Geometry check sheet. Reference: the model listing, model coordinates, mm. Face numbers are marked on the shaded views. Round coordinates to 2 decimals unless told otherwise and drop trailing zeros. Order: outer loops, then holes, each group sorted by start corner. A loop starts at its lowest first (then second) coordinate and runs counter-clockwise, first axis right, second up.
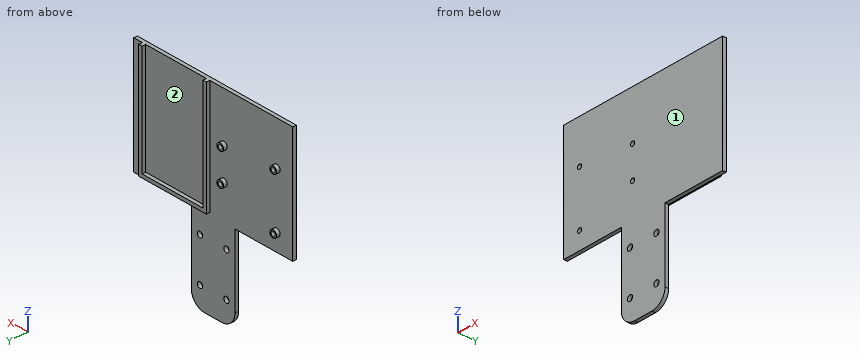
```python
from build123d import *

# Parameters (mm, degrees)
SKETCH1_W           = 41.91
SKETCH1_H           = 76.2
SKETCH1_R           = 2.54
BOSS_EXTRUDE1_DEPTH = 3.175
SKETCH2_W           = 152.4
SKETCH2_H           = 101.6
BOSS_EXTRUDE2_DEPTH = 3.175
SKETCH3_R           = 2
CUT_EXTRUDE1_DEPTH  = 160.162214816
BOSS_EXTRUDE3_DEPTH = 3.175
BOSS_EXTRUDE4_START = 3.175
SKETCH5_R           = 3.175
SKETCH5_R_2         = 2
BOSS_EXTRUDE4_DEPTH = 3.175
FILLET1_R           = 12.7


with BuildPart() as part:
    # Sketch1 → Boss-Extrude1 (new body)
    with BuildSketch(Plane(origin=(0, 0, 0), x_dir=(1, 0, 0), z_dir=(0, 1, 0))):
        Rectangle(SKETCH1_W, SKETCH1_H)
        with Locations(Location((-12.7, 19.05, 0), (0, 0, 270))):
            Circle(SKETCH1_R, mode=Mode.SUBTRACT)
        with Locations(Location((-12.7, -19.05, 0), (0, 0, 270))):
            Circle(SKETCH1_R, mode=Mode.SUBTRACT)
        with Locations(Location((12.7, -19.05, 0), (0, 0, 270))):
            Circle(SKETCH1_R, mode=Mode.SUBTRACT)
        with Locations(Location((12.7, 19.05, 0), (0, 0, 270))):
            Circle(SKETCH1_R, mode=Mode.SUBTRACT)
    extrude(amount=BOSS_EXTRUDE1_DEPTH)

    # Sketch2 → Boss-Extrude2 (add)
    with BuildSketch(Plane(origin=(0, 3.175, 0), x_dir=(1, 0, 0), z_dir=(0, 1, 0))):
        with Locations((0, -88.9)):
            Rectangle(SKETCH2_W, SKETCH2_H)
    extrude(amount=-BOSS_EXTRUDE2_DEPTH)

    # Sketch3 → Cut-Extrude1 (cut, through all)
    with BuildSketch(Plane(origin=(0, 3.175, 0), x_dir=(1, 0, 0), z_dir=(0, 1, 0))):
        with Locations(Location((-60.96, -53.34, 0), (0, 0, 270))):
            Circle(SKETCH3_R)
        with Locations(Location((-60.96, -101.6, 0), (0, 0, 270))):
            Circle(SKETCH3_R)
        with Locations(Location((-10.16, -68.58, 0), (0, 0, 270))):
            Circle(SKETCH3_R)
        with Locations(Location((-10.16, -96.52, 0), (0, 0, 270))):
            Circle(SKETCH3_R)
    extrude(amount=-CUT_EXTRUDE1_DEPTH, mode=Mode.SUBTRACT)

    # Sketch4 → Boss-Extrude3 (add)
    with BuildSketch(Plane(origin=(0, 3.175, 0), x_dir=(1, 0, 0), z_dir=(0, 1, 0))):
        Polygon((64.77, -43.18), (64.77, -120.65), (64.77, -139.7), (67.945, -139.7), (67.945, -120.65), (67.945, -40.005), (3.175, -40.005), (3.175, -120.65), (3.175, -139.7), (6.35, -139.7), (6.35, -120.65), (6.35, -43.18), align=None)
    extrude(amount=BOSS_EXTRUDE3_DEPTH)

    # Sketch5 → Boss-Extrude4 (add)
    # profile 1 of 4: a face of its own
    with BuildSketch(Plane(origin=(0, 3.175, 0), x_dir=(1, 0, 0), z_dir=(0, 1, 0)).offset(BOSS_EXTRUDE4_START)):
        with Locations(Location((-60.96, -53.34, 0), (0, 0, 90))):
            Circle(SKETCH5_R)
        with Locations(Location((-60.96, -53.34, 0), (0, 0, 270))):
            Circle(SKETCH5_R_2, mode=Mode.SUBTRACT)
    # profile 2 of 4: a face of its own
    with BuildSketch(Plane(origin=(0, 3.175, 0), x_dir=(1, 0, 0), z_dir=(0, 1, 0)).offset(BOSS_EXTRUDE4_START)):
        with Locations(Location((-60.96, -101.6, 0), (0, 0, 90))):
            Circle(SKETCH5_R)
        with Locations(Location((-60.96, -101.6, 0), (0, 0, 270))):
            Circle(SKETCH5_R_2, mode=Mode.SUBTRACT)
    # profile 3 of 4: a face of its own
    with BuildSketch(Plane(origin=(0, 3.175, 0), x_dir=(1, 0, 0), z_dir=(0, 1, 0)).offset(BOSS_EXTRUDE4_START)):
        with Locations(Location((-10.16, -96.52, 0), (0, 0, 90))):
            Circle(SKETCH5_R)
        with Locations(Location((-10.16, -96.52, 0), (0, 0, 270))):
            Circle(SKETCH5_R_2, mode=Mode.SUBTRACT)
    # profile 4 of 4: a face of its own
    with BuildSketch(Plane(origin=(0, 3.175, 0), x_dir=(1, 0, 0), z_dir=(0, 1, 0)).offset(BOSS_EXTRUDE4_START)):
        with Locations(Location((-10.16, -68.58, 0), (0, 0, 90))):
            Circle(SKETCH5_R)
        with Locations(Location((-10.16, -68.58, 0), (0, 0, 270))):
            Circle(SKETCH5_R_2, mode=Mode.SUBTRACT)
    extrude(amount=-BOSS_EXTRUDE4_DEPTH)

    # Fillet1
    fillet1_edges = [part.edges().sort_by_distance(p)[0] for p in [
        (-20.955, 1.5875, -38.1),
        (20.955, 1.5875, -38.1),
    ]]
    fillet(fillet1_edges, radius=FILLET1_R)


solid = part.part
```
(1) Sectioned sample at D-D, the plane x = 12.7. Record the cut outline in (y, z) (3 decimals).
Returned:
outline: (0, -37.297) - (3.175, -37.297) - (3.175, -21.59) - (0, -21.59) - close; (0, -16.51) - (3.175, -16.51) - (3.175, 16.51) - (0, 16.51) - close; (0, 21.59) - (3.175, 21.59) - (3.175, 40.005) - (6.35, 40.005) - (6.35, 43.18) - (3.175, 43.18) - (3.175, 139.7) - (0, 139.7) - close
(2) Sectioned sample at C-C, the plane x = 61. Record the cut outline in (y, z) (3 decimals), and give its area (3 significant figures).
Returned:
outline: (0, 38.1) - (3.175, 38.1) - (3.175, 40.005) - (6.35, 40.005) - (6.35, 43.18) - (3.175, 43.18) - (3.175, 139.7) - (0, 139.7) - close
area: 333 mm2
(3) Material ranges on line 1 (X direction, y = 4, z = 101.6) (3 decimals); line 2 (X direction, y = 2.2, z = 19.05) (3 decimals); line 3 (X direction, y = 5, z = 131.5) (3 decimals), recorded low to high.
Returned:
line 1: x = -64.135 to -62.96, -58.96 to -57.785, 3.175 to 6.35, 64.77 to 67.945
line 2: x = -20.955 to -15.24, -10.16 to 10.16, 15.24 to 20.955
line 3: x = 3.175 to 6.35, 64.77 to 67.945
(4) Sectioned sample at B-B, the plane z = 19.05. Record the cut outline in (x, y) (3 decimals), and give its area (3 significant figures).
Returned:
outline: (-20.955, 0) - (-15.24, 0) - (-15.24, 3.175) - (-20.955, 3.175) - close; (-10.16, 0) - (10.16, 0) - (10.16, 3.175) - (-10.16, 3.175) - close; (15.24, 0) - (20.955, 0) - (20.955, 3.175) - (15.24, 3.175) - close
area: 101 mm2
(5) Draft check along X on the marked faces 1 and 2. Enter one of: released by +X, released by -X, zero draft, split by the parting line, or undercut.
Returned:
face 1: zero draft
face 2: undercut
(6) Sectioned sample at A-A, the plane z = 53.34. Record the cut outline in (x, y) (3 decimals).
Returned:
outline: (-76.2, 0) - (-62.96, 0) - (-62.96, 6.35) - (-64.135, 6.35) - (-64.135, 3.175) - (-76.2, 3.175) - close; (-58.96, 0) - (76.2, 0) - (76.2, 3.175) - (67.945, 3.175) - (67.945, 6.35) - (64.77, 6.35) - (64.77, 3.175) - (6.35, 3.175) - (6.35, 6.35) - (3.175, 6.35) - (3.175, 3.175) - (-57.785, 3.175) - (-57.785, 6.35) - (-58.96, 6.35) - close
(7) Depth check by flat-ended pin: P1, Ø5, axis at x = -60.96, z = 53.34, coming from the -Y side; P2, Ø8, axis at x = 13.5, z = 61.5, coming from the +Y side (3 decimals); P3, Ø3.5, axis at x = 21, y = 5, coming from the +Z side; P4, Ø1, axis at x = 58, y = 1.5, coming from the -Z side. Enter the tip coordinate at first touch or a pass-through.
Returned:
P1: stops at y = 0
P2: stops at y = 3.175
P3: stops at z = 43.18
P4: stops at z = 38.1
